Check sheet for the modelled part. Datum: model origin and axes. Units: mm. Round coordinates to 2 decimals unless told otherwise and drop trailing zeros. Write each loop counter-clockwise with the first axis right and the second up, starting at its lowest first coordinate (ties: lowest second). Pieces come first, ordered by that corner, then holes.
Item 1: Section check A-A, the plane x = -41. Record the cut outline in (y, z).
Item 2: Section check C-C, the plane z = 0.45. State how many separate pieces and enclosed holes the cut face has, plus the area to 3 significant figures.
Item 3: Section check B-B, the plane y = -20.5. Record the cut outline in (x, z), plus the area to 3 significant figures.
Item 4: Section check D-D, the plane x = 3. Record the cut outline in (y, z).
Item 5: Depth check by flat-ended pin: pin 1 (0.9 mm diameter, centred on y = -30.5, z = 1, fed in from +X); pin 2 (0.9 mm diameter, centred on x = -63, z = 1, fed in from -Y); pin 3 (1.5 mm diameter, centred on x = -71, z = 1.5, fed in from -Y). Enter the tip coordinate at first touch or a pass-through.
Item 6: Material ranges on line 1 along Y through (x, z) = (-45, 1.6); line 2 along X through (y, z) = (-15.5, 1.4); line 3 along X through (y, z) = (-24.5, 2.1), recorded low to high.
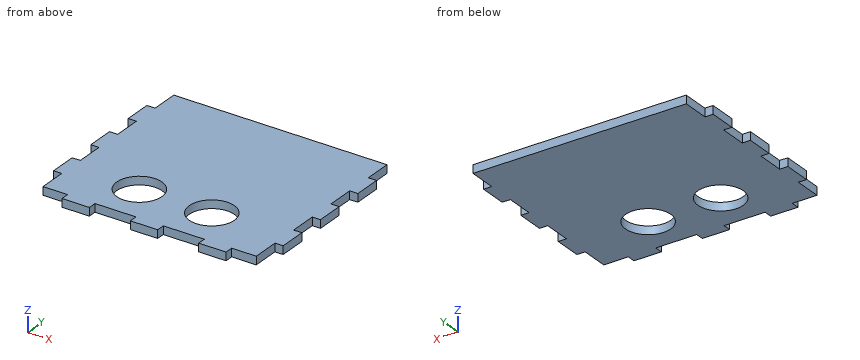
from build123d import *

# Parameters (mm, degrees)
ESQUISSE1_R        = 8.25
BOSS_EXTRU_1_DEPTH = 3


with BuildPart() as part:
    # Esquisse1 → Boss.-Extru.1 (new body)
    with BuildSketch(Plane.XY):
        Polygon((-69.538481563, 40.597826087), (8.461518437, 40.597826087), (8.461518437, 30.597826087), (11.461518437, 30.597826087), (11.461518437, 20.597826087), (8.461518437, 20.597826087), (8.461518437, 10.597826087), (11.461518437, 10.597826087), (11.461518437, 0.597826087), (8.461518437, 0.597826087), (8.461518437, -9.402173913), (11.461518437, -9.402173913), (11.461518437, -19.402173913), (8.461518437, -19.402173913), (8.461518437, -29.402173913), (-0.538481563, -29.402173913), (-0.538481563, -32.402173913), (-10.538481563, -32.402173913), (-10.538481563, -29.402173913), (-25.538481563, -29.402173913), (-25.538481563, -32.402173913), (-35.538481563, -32.402173913), (-35.538481563, -29.402173913), (-50.538481563, -29.402173913), (-50.538481563, -32.402173913), (-60.538481563, -32.402173913), (-60.538481563, -29.402173913), (-69.538481563, -29.402173913), (-69.538481563, -19.402173913), (-72.538481563, -19.402173913), (-72.538481563, -9.402173913), (-69.538481563, -9.402173913), (-69.538481563, 0.597826087), (-72.538481563, 0.597826087), (-72.538481563, 10.597826087), (-69.538481563, 10.597826087), (-69.538481563, 20.597826087), (-72.538481563, 20.597826087), (-72.538481563, 30.597826087), (-69.538481563, 30.597826087), align=None)
        with Locations((-18.038481563, -14.402173913)):
            Circle(ESQUISSE1_R, mode=Mode.SUBTRACT)
        with Locations((-44.538481563, -14.402173913)):
            Circle(ESQUISSE1_R, mode=Mode.SUBTRACT)
    extrude(amount=BOSS_EXTRU_1_DEPTH)


solid = part.part
Values found:
1. outline: (-29.4, 0) - (-21.85, 0) - (-21.85, 3) - (-29.4, 3) - close; (-6.95, 0) - (40.6, 0) - (40.6, 3) - (-6.95, 3) - close
2. separate pieces: 1
2. enclosed holes: 2
2. area: 5,300 mm2
3. outline: (-69.54, 0) - (-50.1, 0) - (-50.1, 3) - (-69.54, 3) - close; (-38.98, 0) - (-23.6, 0) - (-23.6, 3) - (-38.98, 3) - close; (-12.48, 0) - (8.46, 0) - (8.46, 3) - (-12.48, 3) - close
3. area: 167 mm2
4. outline: (-29.4, 0) - (40.6, 0) - (40.6, 3) - (-29.4, 3) - close
5. pin 1: stops at x = -0.54
5. pin 2: stops at y = -29.4
5. pin 3: stops at y = -19.4
6. line 1: y = -29.4 to -22.64, -6.17 to 40.6
6. line 2: x = -72.54 to -52.72, -36.36 to -26.22, -9.86 to 11.46
6. line 3: x = -69.54 to 8.46
